Check sheet for the modelled part. Datum: model origin and axes. Units: mm. Round coordinates to 2 decimals unless told otherwise and drop trailing zeros. Write each loop counter-clockwise with the first axis right and the second up, starting at its lowest first coordinate (ties: lowest second). Pieces come first, ordered by that corner, then holes.
Item 1: Material ranges on line 1 along Y through (x, z) = (0, 5.75); line 2 along X through (y, z) = (-2.5, 5.5); line 3 along X through (y, z) = (4.75, 6), recorded low to high.
Item 2: Section check A-A, the plane z = -1.5. Record the cut outline in (x, y).
Item 3: Release check for a two-part mould opening along X. For faces 1 (the flat face through (-8, 10, 0)), 2 (the cylindrical face through (5.72, -11, -1.68)), 3 (the cylindrical face through (-0.853, 6.494, 2.319)) record: pulls with the +X half, pulls with the -X half, needs draft (parallel to the pull), parting line crosses it, or undercut.
Item 4: Depth check by flat-ended pin: pin 1 (3 mm diameter, centred on x = 11.5, z = 6, fed in from -Y); pin 2 (5 mm diameter, centred on y = -5.5, z = 5.5, fed in from +X); pin 3 (3 mm diameter, centred on x = 7, z = 2.5, fed in from +Y). Enter the tip coordinate at first touch or a pass-through.
from build123d import *

# Parameters (mm, degrees)
F0_R        = 12.4
F0_R_2      = 6.55
F1_DEPTH    = 3.4
F0_R_3      = 14.75
F1_FACE_R   = 12.4
F1_FACE_R_2 = 6.55
F2_DEPTH    = 8.2
F3_R        = 8.19999


# Not quite as in the source:
# - a fillet or chamfer is up to 0.001 mm smaller than in the source, because OpenCascade refuses the exact size


with BuildPart() as f1:
    # F0 (on Top) → F1 (new body)
    with BuildSketch(Plane.XY):
        Circle(F0_R)
        Circle(F0_R_2, mode=Mode.SUBTRACT)
    extrude(amount=-F1_DEPTH)

    # F0 (on Top) + F1_face (on face) → F2 (join)
    with BuildSketch(Plane.XY):
        Circle(F0_R_3)
        Circle(F0_R, mode=Mode.SUBTRACT)
    with BuildSketch(Plane.XY):
        Circle(F1_FACE_R)
        Circle(F1_FACE_R_2, mode=Mode.SUBTRACT)
    extrude(amount=F2_DEPTH)

    # F3 (radius 8.2 in the source; OpenCascade refuses exactly that, so slightly less here)
    f3_edges = [f1.edges().sort_by_distance(p)[0] for p in [
        (-14.75, 0, 8.2),
    ]]
    fillet(f3_edges, radius=F3_R)


solid = f1.part
Values found:
1. line 1: y = -12.4 to -6.55, 6.55 to 12.4
1. line 2: x = -12.38 to -6.05, 6.05 to 12.38
1. line 3: x = -11.17 to -4.51, 4.51 to 11.17
2. outline: circle Ø24.8 at (0, 0); hole circle Ø13.1 at (0, 0)
3. face 1: needs draft
3. face 2: parting line crosses it
3. face 3: undercut
4. pin 1: stops at y = -7.91
4. pin 2: stops at x = 13.39
4. pin 3: stops at y = 13.4
